```python
from build123d import *

# Parameters (mm, degrees)
F1_DEPTH  = 40
F2_T      = -2.5
F3_W      = 40
F3_H      = 10
F4_DEPTH  = 5
F5_W      = 40
F5_H      = 10
F6_DEPTH  = 5
F8_DEPTH  = 45.001
F10_DEPTH = 45.001


with BuildPart() as f1:
    # F0 (on Top) → F1 (new body)
    with BuildSketch(Plane.XY):
        Polygon((4, 40), (0, 40), (0, 0), (40, 0), (40, 4), align=None)
    extrude(amount=F1_DEPTH)

    # F2
    f2_openings = [f1.faces().sort_by_distance(p)[0] for p in [
        (22, 22, 20),
    ]]
    offset(amount=F2_T, openings=f2_openings)

    # F3 (on face) → F4 (join)
    with BuildSketch(Plane(origin=(0, 0, 0), x_dir=(0, -1, 0), z_dir=(-1, 0, 0))):
        with Locations((-20, 20)):
            Rectangle(F3_W, F3_H)
    extrude(amount=F4_DEPTH)

    # F5 (on face) → F6 (join)
    with BuildSketch(Plane.XZ):
        with Locations((20, 20)):
            Rectangle(F5_W, F5_H)
    extrude(amount=F6_DEPTH)

    # F7 (on face) → F8 (cut, through all)
    with BuildSketch(Plane.XZ.offset(5)):
        with BuildLine():
            Line((27.5, 24), (12.5, 24))
            ThreePointArc((12.5, 24), (8.5, 20), (12.5, 16))
            Line((12.5, 16), (27.5, 16))
            ThreePointArc((27.5, 16), (31.5, 20), (27.5, 24))
        make_face()
    extrude(amount=-F8_DEPTH, mode=Mode.SUBTRACT)

    # F9 (on face) → F10 (cut, through all)
    with BuildSketch(Plane(origin=(-5, 0, 0), x_dir=(0, -1, 0), z_dir=(-1, 0, 0))):
        with BuildLine():
            ThreePointArc((-27.5, 24), (-31.5, 20), (-27.5, 16))
            Line((-27.5, 16), (-12.5, 16))
            ThreePointArc((-12.5, 16), (-8.5, 20), (-12.5, 24))
            Line((-12.5, 24), (-27.5, 24))
        make_face()
    extrude(amount=-F10_DEPTH, mode=Mode.SUBTRACT)


solid = f1.part
```
CAD build for the part. Positions are in the model's coordinates, mm. A direction names the side the tool comes from. Give positions to 0.01 mm unless a question says otherwise; leave off trailing zeros. Write each loop counter-clockwise with the first axis right and the second up, starting at its lowest first coordinate (ties: lowest second). Pieces come first, ordered by that corner, then holes. Notation, with made-up numbers: (25.25, 85.25) -> (70.25, 85.25) arc R22 cw to (70.25, 96.25) -> close; hole circle Ø8 at (86, 10). An arc over 180 degrees is marked (long way). Write each question's results on one line, items separated by ' | '.
1. Cut at C-C, the plane z = 23. Write the cut outline in (x, y).
Geometry check:
outline: (-5, 0) -> (0, 0) -> (0, -5) -> (9.85, -5) -> (9.85, 2.5) -> (2.5, 2.5) -> (2.5, 9.85) -> (-5, 9.85) -> close; (-5, 30.15) -> (2.5, 30.15) -> (2.5, 37.5) -> (6.5, 37.5) -> (4, 40) -> (-5, 40) -> close; (30.15, -5) -> (40, -5) -> (40, 4) -> (37.5, 6.5) -> (37.5, 2.5) -> (30.15, 2.5) -> close
2. Wall check: probe 1 along Z at (x, y) = (12, 20); probe 2 along Y at (x, z) = (17, 9); probe 3 along Y at (x, z) = (-3, 20.5). Give the ranges that are in metal, low to high. Write a range as [from, to].
Geometry check:
probe 1: [0, 2.5], [37.5, 40] | probe 2: [0, 2.5] | probe 3: [0, 8.53], [31.47, 40]
3. Cut at B-B, the plane x = 20. Write the cut outline in (y, z), then the cut area to 4 significant figures.
Geometry check:
outline: (-5, 15) -> (0, 15) -> (0, 0) -> (24, 0) -> (24, 2.5) -> (2.5, 2.5) -> (2.5, 16) -> (-5, 16) -> close; (-5, 24) -> (2.5, 24) -> (2.5, 37.5) -> (24, 37.5) -> (24, 40) -> (0, 40) -> (0, 25) -> (-5, 25) -> close | area: 197.5 mm²
4. Cut at A-A, the plane y = 17. Write the cut outline in (x, z).
Geometry check:
outline: (-5, 15) -> (0, 15) -> (0, 0) -> (27, 0) -> (27, 2.5) -> (2.5, 2.5) -> (2.5, 16) -> (-5, 16) -> close; (-5, 24) -> (2.5, 24) -> (2.5, 37.5) -> (27, 37.5) -> (27, 40) -> (0, 40) -> (0, 25) -> (-5, 25) -> close
5. Cut at D-D, the plane z = 28. Write the cut outline in (x, y).
Geometry check:
outline: (0, 0) -> (40, 0) -> (40, 4) -> (37.5, 6.5) -> (37.5, 2.5) -> (2.5, 2.5) -> (2.5, 37.5) -> (6.5, 37.5) -> (4, 40) -> (0, 40) -> close
6. Two-plate mould, pull along Y, no slides. Class faces 4 (the flat face through (22, 22, 2)), 5 (the flat face through (0, 20, 32)), 6 (the flat face through (5, 37.5, 20)): pulls with the +Y half, pulls with the -Y half, needs draft (parallel to the pull), parting line crosses it, or undercut.
Geometry check:
face 4: pulls with the +Y half | face 5: needs draft | face 6: undercut
7. Drop flat-ended pins along their axis: P1, Ø3, axis at x = 3.5, z = 4, coming from the -Y side; P2, Ø16.5, axis at y = 12.5, z = 30, coming from the -X side; P3, Ø1, axis at y = 22, z = 30, coming from the +X side; P4, Ø4, axis at x = -2.5, y = 23.5, coming from the +Z side. Give the stop position or say it passes through.
Geometry check:
P1: y = 0 | P2: x = -5 | P3: x = 2.5 | P4: z = 25
8. Which spindle directions (+Z, -Z, +X, -X, +Y, -Y) get a long thin tool onto all of the face, cutting with end or side? Do faces 1 (the flat face through (0, -2, 20)), 2 (the cylindrical face through (8.5, -1.3, 20.1)), 3 (the flat face through (20, -2, 15)). Say none if no direction does.
Geometry check:
face 1: +Z, -Z, -X, -Y | face 2: +Y, -Y | face 3: -Z, +X, -X, -Y
